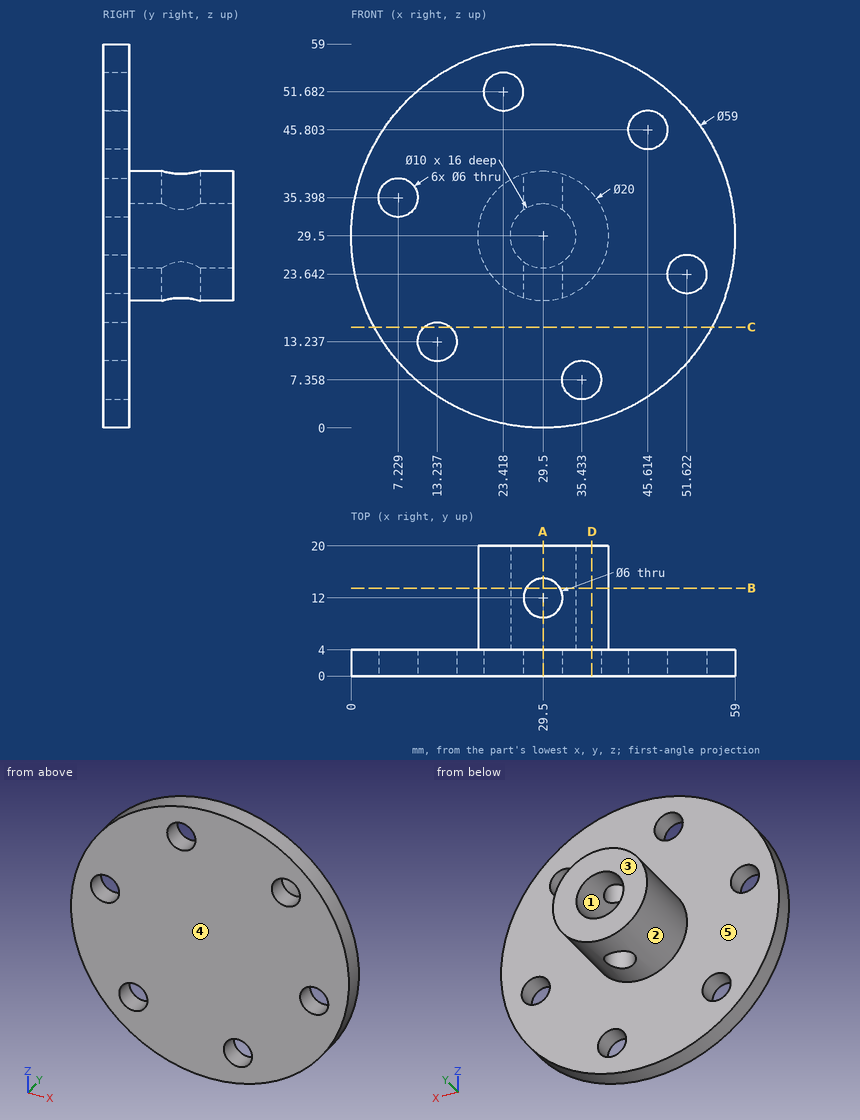
Answer from the drawing. Dimensions are ordinates in mm from the lowest x, y and z of the part. A direction names the side the tool comes from. Give positions to 0.01 mm unless a question says otherwise; leave off trailing zeros. Write each loop counter-clockwise with the first axis right and the second up, starting at its lowest first coordinate (ties: lowest second). Pieces come first, ordered by that corner, then holes. Notation, with made-up numbers: (31, 42.25) -> (85, 42.25) arc R26 ccw to (85, 60.25) -> close; hole circle Ø1 at (-25, 47). An arc over 180 degrees is marked (long way). Use a Markdown table: item, result.
(1) Section B-B, the plane y = 13.5 is taken. Determine the outline of the cut face in (x, z), then the cut area to 3 significant figures.
Return value:
| item | result |
|---|---|
| outline | (26.9, 19.84) -> (26.9, 25.23) arc R5 cw to (26.9, 33.77) -> (26.9, 39.16) arc R10 ccw to start; (32.1, 19.84) arc R10 ccw to (32.1, 39.16) -> (32.1, 33.77) arc R5 cw to (32.1, 25.23) -> close |
| area | 182 mm2 |
(2) Section C-C, the plane z = 15.5 is taken. Determine the outline of the cut face in (x, y) (1 decimal), then the cut area to 3 significant figures.
Return value:
| item | result |
|---|---|
| outline | (3.5, 0) -> (11.3, 0) -> (11.3, 4) -> (3.5, 4) -> close; (15.2, 0) -> (55.5, 0) -> (55.5, 4) -> (15.2, 4) -> close |
| area | 192 mm2 |
(3) Flat-ended cylindrical pins translate along their axes: P1, Ø8, axis at x = 29.5, y = 12, coming from the -Z side; P2, Ø3, axis at x = 31, z = 29, coming from the +Y side; P3, Ø5, axis at x = 50, y = 6, coming from the -Z side (1 decimal). Find the tip coordinate at first contact, or state that the pin passes through.
Return value:
| item | result |
|---|---|
| P1 | z = 19.5 |
| P2 | y = 4 |
| P3 | z = 6.9 |
(4) Determine the mould class of the marked faces 1, 2 and 3 for opening direction X: released by +X, released by -X, zero draft, split by the parting line, or undercut.
Return value:
| item | result |
|---|---|
| face 1 | undercut |
| face 2 | split by the parting line |
| face 3 | zero draft |
(5) Find the intervals of material crossed by probe 1 along X at (y, z) = (7.25, 29.5); probe 2 along Y at (x, z) = (12, 34.5); probe 3 along X at (y, z) = (8.5, 28), in increasing order. Write a range as from..to.
Return value:
| item | result |
|---|---|
| probe 1 | 19.5..24.5, 34.5..39.5 |
| probe 2 | 0..4 |
| probe 3 | 19.61..24.73, 34.27..39.39 |
(6) Section D-D, the plane x = 37 is taken. Determine the outline of the cut face in (y, z) (1 decimal).
Return value:
| item | result |
|---|---|
| outline | (0, 1) -> (4, 1) -> (4, 4.8) -> (0, 4.8) -> close; (0, 9.9) -> (4, 9.9) -> (4, 22.9) -> (20, 22.9) -> (20, 36.1) -> (4, 36.1) -> (4, 58) -> (0, 58) -> close |
(7) Section A-A, the plane x = 29.5 is taken. Determine the outline of the cut face in (y, z), then the cut area to 3 significant figures.
Return value:
| item | result |
|---|---|
| outline | (0, 0) -> (4, 0) -> (4, 19.5) -> (9, 19.5) -> (9, 24.5) -> (4, 24.5) -> (4, 34.5) -> (9, 34.5) -> (9, 39.5) -> (4, 39.5) -> (4, 59) -> (0, 59) -> close; (15, 19.5) -> (20, 19.5) -> (20, 24.5) -> (15, 24.5) -> close; (15, 34.5) -> (20, 34.5) -> (20, 39.5) -> (15, 39.5) -> close |
| area | 336 mm2 |
(8) For the marked faces 4 and 5, determine the directions among +Z, -Z, +X, -X, +Y, -Y from which every point of the face is accessible in a straight line to the end or side of a thin tool.
Return value:
| item | result |
|---|---|
| face 4 | +Z, -Z, +X, -X, -Y |
| face 5 | +Y |
